Design review of the part built by this model. Coordinates are the model's own, in mm. A direction names the side the tool comes from. Coordinates: 2 decimals unless noted, no trailing zeros. Write each loop counter-clockwise with the first axis right and the second up, starting at its lowest first coordinate (ties: lowest second). Pieces come first, ordered by that corner, then holes. Notation, with made-up numbers: (40.25, 23.5) - (58.25, 23.5) arc R14 ccw to (58.25, 39.5) - close; hole circle Ø11 at (-30.5, 83). An arc over 180 degrees is marked (long way). Use a Markdown table: item, result.
from build123d import *

# Parameters (mm, degrees)
IZIM1_W                          = 78
IZIM1_H                          = 400
Y_KSEKLIK_EKSTR_ZYON1_DEPTH      = 15
IZIM2_R                          = 25
KES_EKSTR_ZYON1_DEPTH            = 30
Y_KSEKLIK_EKSTR_ZYON2_DEPTH      = 85
Y_KSEKLIK_EKSTR_ZYON2_DEPTH_BACK = 163
IZIM3_W                          = 15
IZIM3_H                          = 15
KES_EKSTR_ZYON2_DEPTH            = 26
IZIM5_W                          = 6
IZIM5_H                          = 6
Y_KSEKLIK_EKSTR_ZYON3_DEPTH      = 65
IZIM6_R                          = 7
KES_EKSTR_ZYON3_DEPTH            = 65
IZIM8_W                          = 72
IZIM8_H                          = 3
Y_KSEKLIK_EKSTR_ZYON4_DEPTH      = 150
IZIM9_W                          = 10
IZIM9_H                          = 5
Y_KSEKLIK_EKSTR_ZYON5_DEPTH      = 5
IZIM12_W                         = 5
IZIM12_H                         = 10
Y_KSEKLIK_EKSTR_ZYON6_DEPTH      = 5
Y_KSEKLIK_EKSTR_ZYON7_DEPTH      = 10
Y_KSEKLIK_EKSTR_ZYON8_DEPTH      = 10
IZIM15_R                         = 2
KES_EKSTR_ZYON5_DEPTH            = 46
RADYUS1_R                        = 2.4
RADYUS2_R                        = 2.4
RADYUS3_R                        = 2.4
RADYUS4_R                        = 2.4


with BuildPart() as part:
    # Çizim1 → Yükseklik-Ekstrüzyon1 (new body)
    with BuildSketch(Plane.XY):
        with Locations((39, -200)):
            Rectangle(IZIM1_W, IZIM1_H)
    extrude(amount=Y_KSEKLIK_EKSTR_ZYON1_DEPTH)

    # Çizim2 → Kes-Ekstrüzyon1 (cut)
    with BuildSketch(Plane.XY.offset(15)):
        with Locations((39, -60)):
            Circle(IZIM2_R)
    extrude(amount=-KES_EKSTR_ZYON1_DEPTH, mode=Mode.SUBTRACT)

    # Çizim3 → Yükseklik-Ekstrüzyon2 (add, two sides: drawn at the far end of the back side and taken through both)
    with BuildSketch(Plane.ZY.offset(-Y_KSEKLIK_EKSTR_ZYON2_DEPTH_BACK)):
        with Locations((7.5, -200)):
            Rectangle(IZIM3_W, IZIM3_H)
        with Locations((7.5, -100)):
            Rectangle(IZIM3_W, IZIM3_H)
        with Locations((7.5, -300)):
            Rectangle(IZIM3_W, IZIM3_H)
    extrude(amount=Y_KSEKLIK_EKSTR_ZYON2_DEPTH + Y_KSEKLIK_EKSTR_ZYON2_DEPTH_BACK)

    # Çizim4 → Kes-Ekstrüzyon2 (cut)
    with BuildSketch(Plane.XY.offset(15)):
        Polygon((24, -261.99590857), (24, -361.99590857), (39, -361.99590857), (54, -361.99590857), (54, -261.99590857), align=None)
    extrude(amount=-KES_EKSTR_ZYON2_DEPTH, mode=Mode.SUBTRACT)

    # Çizim5 → Yükseklik-Ekstrüzyon3 (add)
    with BuildSketch(Plane.XY.offset(15)):
        Polygon((75, -3), (78, -3), (78, -156), (0, -156), (0, -3), (3, -3), (3, -153), (75, -153), align=None)
        with Locations((3, -397)):
            Rectangle(IZIM5_W, IZIM5_H)
        with Locations((75, -397)):
            Rectangle(IZIM5_W, IZIM5_H)
    extrude(amount=Y_KSEKLIK_EKSTR_ZYON3_DEPTH)

    # Çizim6 → Kes-Ekstrüzyon3 (cut)
    with BuildSketch(Plane(origin=(0, 0, 0), x_dir=(-1, 0, 0), z_dir=(0, 0, -1))):
        with Locations((-39, -140)):
            Circle(IZIM6_R)
    extrude(amount=-KES_EKSTR_ZYON3_DEPTH, mode=Mode.SUBTRACT)

    # Çizim8 → Yükseklik-Ekstrüzyon4 (add)
    with BuildSketch(Plane(origin=(0, -153, 0), x_dir=(1, 0, 0), z_dir=(0, 1, 0))):
        with Locations((39, -78.5)):
            Rectangle(IZIM8_W, IZIM8_H)
    extrude(amount=Y_KSEKLIK_EKSTR_ZYON4_DEPTH)

    # Çizim9 → Yükseklik-Ekstrüzyon5 (add)
    with BuildSketch(Plane.ZY):
        with Locations((60, -5.5)):
            Rectangle(IZIM9_W, IZIM9_H)
        with Locations((30, -5.5)):
            Rectangle(IZIM9_W, IZIM9_H)
    extrude(amount=Y_KSEKLIK_EKSTR_ZYON5_DEPTH)

    # Çizim12 → Yükseklik-Ekstrüzyon6 (add)
    with BuildSketch(Plane(origin=(0, -3, 0), x_dir=(1, 0, 0), z_dir=(0, 1, 0))):
        with Locations((-2.5, -30)):
            Rectangle(IZIM12_W, IZIM12_H)
        with Locations((-2.5, -60)):
            Rectangle(IZIM12_W, IZIM12_H)
    extrude(amount=Y_KSEKLIK_EKSTR_ZYON6_DEPTH)

    # Çizim13 → Yükseklik-Ekstrüzyon7 (add)
    with BuildSketch(Plane.XY.offset(65)):
        Polygon((-5, -8), (0, -8), (0, -13), align=None)
    extrude(amount=-Y_KSEKLIK_EKSTR_ZYON7_DEPTH)

    # Çizim14 → Yükseklik-Ekstrüzyon8 (add)
    with BuildSketch(Plane(origin=(0, 0, 25), x_dir=(-1, 0, 0), z_dir=(0, 0, -1))):
        Polygon((0, -8), (0, -13), (5, -8), align=None)
    extrude(amount=-Y_KSEKLIK_EKSTR_ZYON8_DEPTH)

    # Çizim15 → Kes-Ekstrüzyon5 (cut)
    with BuildSketch(Plane(origin=(0, 0, 25), x_dir=(-1, 0, 0), z_dir=(0, 0, -1))):
        with Locations((2.5, -0.5)):
            Circle(IZIM15_R)
    extrude(amount=-KES_EKSTR_ZYON5_DEPTH, mode=Mode.SUBTRACT)

    # Radyus1
    radyus1_edges = [part.edges().sort_by_distance(p)[0] for p in [
        (0, 2, 60),
    ]]
    fillet(radyus1_edges, radius=RADYUS1_R)

    # Radyus2
    radyus2_edges = [part.edges().sort_by_distance(p)[0] for p in [
        (0, 2, 30),
    ]]
    fillet(radyus2_edges, radius=RADYUS2_R)

    # Radyus3
    radyus3_edges = [part.edges().sort_by_distance(p)[0] for p in [
        (-5, 2, 30),
    ]]
    fillet(radyus3_edges, radius=RADYUS3_R)

    # Radyus4
    radyus4_edges = [part.edges().sort_by_distance(p)[0] for p in [
        (-5, 2, 60),
    ]]
    fillet(radyus4_edges, radius=RADYUS4_R)


solid = part.part
(1) For pin 1 (4.5 mm diameter, centred on x = 125.5, z = 4, fed in from +Y); pin 2 (1 mm diameter, centred on y = -356.5, z = 11, fed in from +X); pin 3 (16.5 mm diameter, centred on x = 102, z = 5.5, fed in from -Y), all flat-tipped, find the tip position at first contact; note any pin that passes through.
Determined:
| item | result |
|---|---|
| pin 1 | y = -92.5 |
| pin 2 | x = 78 |
| pin 3 | y = -307.5 |
(2) Take a section at C-C on y = -268. Write out the cut boundary in (x, z).
Determined:
| item | result |
|---|---|
| outline | (0, 0) - (24, 0) - (24, 15) - (0, 15) - close; (54, 0) - (78, 0) - (78, 15) - (54, 15) - close |
(3) For L1, parallel to Y at x = 39, z = 10.5; L2, parallel to Y at x = 136.5, z = 6.5; L3, parallel to Z at x = 37.5, y = -87.5, list the stretches that pass through material, from the lowest coordinate up. Write a range as from..to.
Determined:
| item | result |
|---|---|
| L1 | -400..-362, -262..-147, -133..-85, -35..0 |
| L2 | -307.5..-292.5, -207.5..-192.5, -107.5..-92.5 |
| L3 | 0..15, 77..80 |
(4) Take a section at A-A on x = -23. Write out the cut boundary in (y, z).
Determined:
| item | result |
|---|---|
| outline | (-307.5, 0) - (-292.5, 0) - (-292.5, 15) - (-307.5, 15) - close; (-207.5, 0) - (-192.5, 0) - (-192.5, 15) - (-207.5, 15) - close; (-107.5, 0) - (-92.5, 0) - (-92.5, 15) - (-107.5, 15) - close |
(5) Draft analysis for pull direction Z (two halves, no side actions). For faces 1 (the flat face through (40, -95, 15)), 2 (the flat face through (-42, -100, 15)), 3 (the flat face through (78, -251, 7)), state which applies: +Z half, -Z half, draft (parallel to the pull), parting line (faces both ways), or undercut.
Determined:
| item | result |
|---|---|
| face 1 | undercut |
| face 2 | +Z half |
| face 3 | draft |
(6) Machinability: for faces 4 (the flat face through (-42, -307.5, 7)), 5 (the flat face through (121, -292.5, 7)), 6 (the flat face through (-42, -107.5, 7)), 7 (the flat face through (54, -313, 8)), 8 (the flat face through (38, -79, 77)), which of the approach directions +Z, -Z, +X, -X, +Y, -Y give a long, thin tool a straight path to every point of the face, cutting with its end or side? Answer none if there is none.
Determined:
| item | result |
|---|---|
| face 4 | +Z, -Z, -X, -Y |
| face 5 | +Z, -Z, +X |
| face 6 | +Z, -Z, -X |
| face 7 | +Z, -Z |
| face 8 | +Y |
(7) Take a section at D-D on y = -115. Write out the cut boundary in (x, z).
Determined:
| item | result |
|---|---|
| outline | (0, 0) - (78, 0) - (78, 80) - (0, 80) - close; hole (3, 15) - (75, 15) - (75, 77) - (3, 77) - close |
(8) Take a section at B-B on z = 30. Write out the cut boundary in (x, y), and give its area (3 significant figures).
Determined:
| item | result |
|---|---|
| outline | (-5, -8) - (0, -13) - (0, -156) - (78, -156) - (78, -3) - (75, -3) - (75, -153) - (3, -153) - (3, -3) - (0, -3) - (0, -0.4) arc R2.4 ccw to (-2.4, 2) - (-2.6, 2) arc R2.4 ccw to (-5, -0.4) - close; (0, -400) - (6, -400) - (6, -394) - (0, -394) - close; (72, -400) - (78, -400) - (78, -394) - (72, -394) - close; hole circle Ø4 at (-2.5, -0.5) |
| area | 1,250 mm2 |
